```python
from build123d import *

# Parameters (mm, degrees)
SKETCH_W                           = 102
SKETCH_H                           = 105
SKETCH_R                           = 11
SKETCH_R_2                         = 13.5
PAD_DEPTH                          = 20
SKETCH001_W                        = 102
SKETCH001_H                        = 55
POCKET_DEPTH                       = 10
SKETCH002_W                        = 42
SKETCH002_H                        = 42
POCKET001_DEPTH                    = 16
POCKET002_DEPTH                    = 315.493809
POCKET002_LINEARPATTERN_2_DEPTH    = 315.493809
POCKET002_LINEARPATTERN_3_DEPTH    = 315.493809
POCKET002_LINEARPATTERN_4_DEPTH    = 315.493809
LINEARPATTERN001_COUNT             = 2
LINEARPATTERN001_PITCH             = 30
SKETCH004_R                        = 1.6
POCKET003_DEPTH                    = 4.001
CHAMFER_SIZE                       = 5
CHAMFER001_SIZE                    = 10
FILLET_R                           = 20
SKETCH006_R                        = 16
POCKET004_DEPTH                    = 16
SKETCH007_R                        = 3
POCKET005_DEPTH                    = 2
POCKET006_DEPTH                    = 4.001
SKETCH009_W                        = 4
SKETCH009_H                        = 42
POCKET007_DEPTH                    = 16
POCKET008_DEPTH                    = 2
POCKET009_DEPTH                    = 20.001
SKETCH012_R                        = 6.5
POCKET010_DEPTH                    = 8
SKETCH012_LINEARPATTERN002_2_R     = 6.5
POCKET010_LINEARPATTERN002_2_DEPTH = 8
SKETCH012_LINEARPATTERN002_3_R     = 6.5
POCKET010_LINEARPATTERN002_3_DEPTH = 8
LINEARPATTERN003_COUNT             = 3
LINEARPATTERN003_PITCH             = 15


with BuildPart() as part:
    # Sketch → Pad (new body)
    with BuildSketch(Plane.XY):
        with Locations((-14, -27.5)):
            Rectangle(SKETCH_W, SKETCH_H)
        with Locations((2, 0)):
            Circle(SKETCH_R, mode=Mode.SUBTRACT)
        with Locations((-40, 0)):
            Circle(SKETCH_R_2, mode=Mode.SUBTRACT)
    extrude(amount=PAD_DEPTH)

    # Sketch001 (on Face8 of Pad) → Pocket (cut)
    with BuildSketch(Plane.XY.offset(20)):
        with Locations((-14, -52.5)):
            Rectangle(SKETCH001_W, SKETCH001_H)
    extrude(amount=-POCKET_DEPTH, mode=Mode.SUBTRACT)

    # Sketch002 (on Face2 of Pocket) → Pocket001 (cut)
    with BuildSketch(Plane(origin=(0, 0, 0), x_dir=(1, 0, 0), z_dir=(0, 0, -1))):
        with Locations((2, 0)):
            Rectangle(SKETCH002_W, SKETCH002_H)
    extrude(amount=-POCKET001_DEPTH, mode=Mode.SUBTRACT)

    # Sketch003 (on Face2 of Pocket001) → Pocket002 (cut, through all)
    with BuildSketch(Plane(origin=(0, 0, 0), x_dir=(1, 0, 0), z_dir=(0, 0, -1))):
        with BuildLine():
            ThreePointArc((26, 35), (28, 33), (30, 35))
            Line((30, 35), (30, 45))
            ThreePointArc((30, 45), (28, 47), (26, 45))
            Line((26, 35), (26, 45))
        make_face()
    pocket002 = extrude(amount=-POCKET002_DEPTH, mode=Mode.SUBTRACT)

    # Sketch003 LinearPattern 2 → Pocket002 LinearPattern 2 (cut, through all)
    with BuildSketch(Plane(origin=(-28, 0, 0), x_dir=(1, 0, 0), z_dir=(0, 0, -1))):
        with BuildLine():
            ThreePointArc((26, 35), (28, 33), (30, 35))
            Line((30, 35), (30, 45))
            ThreePointArc((30, 45), (28, 47), (26, 45))
            Line((26, 35), (26, 45))
        make_face()
    pocket002_linearpattern_2 = extrude(amount=-POCKET002_LINEARPATTERN_2_DEPTH, mode=Mode.SUBTRACT)

    # Sketch003 LinearPattern 3 → Pocket002 LinearPattern 3 (cut, through all)
    with BuildSketch(Plane(origin=(-56, 0, 0), x_dir=(1, 0, 0), z_dir=(0, 0, -1))):
        with BuildLine():
            ThreePointArc((26, 35), (28, 33), (30, 35))
            Line((30, 35), (30, 45))
            ThreePointArc((30, 45), (28, 47), (26, 45))
            Line((26, 35), (26, 45))
        make_face()
    pocket002_linearpattern_3 = extrude(amount=-POCKET002_LINEARPATTERN_3_DEPTH, mode=Mode.SUBTRACT)

    # Sketch003 LinearPattern 4 → Pocket002 LinearPattern 4 (cut, through all)
    with BuildSketch(Plane(origin=(-84, 0, 0), x_dir=(1, 0, 0), z_dir=(0, 0, -1))):
        with BuildLine():
            ThreePointArc((26, 35), (28, 33), (30, 35))
            Line((30, 35), (30, 45))
            ThreePointArc((30, 45), (28, 47), (26, 45))
            Line((26, 35), (26, 45))
        make_face()
    pocket002_linearpattern_4 = extrude(amount=-POCKET002_LINEARPATTERN_4_DEPTH, mode=Mode.SUBTRACT)

    # LinearPattern001: Pocket002, Pocket002 LinearPattern 2, Pocket002 LinearPattern 3, Pocket002 LinearPattern 4 ×2
    with Locations(*[(0, -i * LINEARPATTERN001_PITCH, 0) for i in range(1, LINEARPATTERN001_COUNT)]):
        add(pocket002, mode=Mode.SUBTRACT)
        add(pocket002_linearpattern_2, mode=Mode.SUBTRACT)
        add(pocket002_linearpattern_3, mode=Mode.SUBTRACT)
        add(pocket002_linearpattern_4, mode=Mode.SUBTRACT)

    # Sketch004 (on Face46 of MultiTransform) → Pocket003 (cut, through all)
    with BuildSketch(Plane(origin=(0, 0, 16), x_dir=(1, 0, 0), z_dir=(0, 0, -1))):
        with Locations((16.5, 15.5)):
            Circle(SKETCH004_R)
        with Locations((16.5, -15.5)):
            Circle(SKETCH004_R)
        with Locations((-14.5, -15.5)):
            Circle(SKETCH004_R)
        with Locations((-14.5, 15.5)):
            Circle(SKETCH004_R)
    extrude(amount=-POCKET003_DEPTH, mode=Mode.SUBTRACT)

    # Chamfer
    chamfer_edges = [part.edges().sort_by_distance(p)[0] for p in [
        (-65, -80, 5),
        (37, -80, 5),
    ]]
    chamfer(chamfer_edges, length=CHAMFER_SIZE)

    # Chamfer001
    chamfer001_edges = [part.edges().sort_by_distance(p)[0] for p in [
        (37, -25, 15),
        (37, 25, 10),
        (-65, -25, 15),
    ]]
    chamfer(chamfer001_edges, length=CHAMFER001_SIZE)

    # Fillet
    fillet_edges = [part.edges().sort_by_distance(p)[0] for p in [
        (-65, 25, 10),
    ]]
    fillet(fillet_edges, radius=FILLET_R)

    # Sketch006 (on Face47 of Fillet) → Pocket004 (cut)
    with BuildSketch(Plane.XY.offset(20)):
        with Locations((-40, 0)):
            Circle(SKETCH006_R)
    extrude(amount=-POCKET004_DEPTH, mode=Mode.SUBTRACT)

    # Sketch007 (on Face47 of Pocket004) → Pocket005 (cut)
    with BuildSketch(Plane.XY.offset(20)):
        with Locations((16.5, 15.5)):
            Circle(SKETCH007_R)
        with Locations((-14.5, 15.5)):
            Circle(SKETCH007_R)
        with Locations((-14.5, -15.5)):
            Circle(SKETCH007_R)
        with Locations((16.5, -15.5)):
            Circle(SKETCH007_R)
    extrude(amount=-POCKET005_DEPTH, mode=Mode.SUBTRACT)

    # Sketch008 (on Face52 of Pocket005) → Pocket006 (cut, through all)
    with BuildSketch(Plane(origin=(0, 0, 16), x_dir=(1, 0, 0), z_dir=(0, 0, -1))):
        with BuildLine():
            ThreePointArc((-14.5, -17.1), (-12.9, -15.5), (-14.5, -13.9))
            Line((-14.5, -13.9), (-16.5, -13.9))
            ThreePointArc((-16.5, -13.9), (-18.1, -15.5), (-16.5, -17.1))
            Line((-14.5, -17.1), (-16.5, -17.1))
        make_face()
        with BuildLine():
            ThreePointArc((-14.5, 13.9), (-12.9, 15.5), (-14.5, 17.1))
            Line((-14.5, 17.1), (-16.5, 17.1))
            ThreePointArc((-16.5, 17.1), (-18.1, 15.5), (-16.5, 13.9))
            Line((-14.5, 13.9), (-16.5, 13.9))
        make_face()
        with BuildLine():
            ThreePointArc((16.5, 13.9), (18.1, 15.5), (16.5, 17.1))
            Line((16.5, 17.1), (14.5, 17.1))
            ThreePointArc((14.5, 17.1), (12.9, 15.5), (14.5, 13.9))
            Line((16.5, 13.9), (14.5, 13.9))
        make_face()
        with BuildLine():
            ThreePointArc((16.5, -17.1), (18.1, -15.5), (16.5, -13.9))
            Line((16.5, -13.9), (14.5, -13.9))
            ThreePointArc((14.5, -13.9), (12.9, -15.5), (14.5, -17.1))
            Line((16.5, -17.1), (14.5, -17.1))
        make_face()
    extrude(amount=-POCKET006_DEPTH, mode=Mode.SUBTRACT)

    # Sketch009 (on Face1 of Pocket006) → Pocket007 (cut)
    with BuildSketch(Plane(origin=(0, 0, 0), x_dir=(1, 0, 0), z_dir=(0, 0, -1))):
        with Locations((-21, 0)):
            Rectangle(SKETCH009_W, SKETCH009_H)
    extrude(amount=-POCKET007_DEPTH, mode=Mode.SUBTRACT)

    # Sketch010 (on Face49 of Pocket007) → Pocket008 (cut)
    with BuildSketch(Plane.XY.offset(20)):
        with BuildLine():
            ThreePointArc((-14.5, 12.5), (-11.5, 15.5), (-14.5, 18.5))
            Line((-14.5, 18.5), (-16.5, 18.5))
            ThreePointArc((-16.5, 18.5), (-19.5, 15.5), (-16.5, 12.5))
            Line((-14.5, 12.5), (-16.5, 12.5))
        make_face()
        with BuildLine():
            ThreePointArc((16.5, 12.5), (19.5, 15.5), (16.5, 18.5))
            Line((16.5, 18.5), (14.5, 18.5))
            ThreePointArc((14.5, 18.5), (11.5, 15.5), (14.5, 12.5))
            Line((16.5, 12.5), (14.5, 12.5))
        make_face()
        with BuildLine():
            ThreePointArc((16.5, -18.5), (19.5, -15.5), (16.5, -12.5))
            Line((16.5, -12.5), (14.5, -12.5))
            ThreePointArc((14.5, -12.5), (11.5, -15.5), (14.5, -18.5))
            Line((16.5, -18.5), (14.5, -18.5))
        make_face()
        with BuildLine():
            ThreePointArc((-14.5, -18.5), (-11.5, -15.5), (-14.5, -12.5))
            Line((-14.5, -12.5), (-16.5, -12.5))
            ThreePointArc((-16.5, -12.5), (-19.5, -15.5), (-16.5, -18.5))
            Line((-14.5, -18.5), (-16.5, -18.5))
        make_face()
    extrude(amount=-POCKET008_DEPTH, mode=Mode.SUBTRACT)

    # Sketch011 (on Face49 of Pocket008) → Pocket009 (cut, through all)
    with BuildSketch(Plane.XY.offset(20)):
        with BuildLine():
            ThreePointArc((0, -11), (11, 0), (0, 11))
            Line((0, 11), (-2, 11))
            ThreePointArc((-2, 11), (-13, 0), (-2, -11))
            Line((0, -11), (-2, -11))
        make_face()
    extrude(amount=-POCKET009_DEPTH, mode=Mode.SUBTRACT)

    # Sketch012 (on Face51 of Pocket009) → Pocket010 (cut)
    with BuildSketch(Plane.XY.offset(10)):
        with Locations((14, -65)):
            Circle(SKETCH012_R)
    pocket010 = extrude(amount=-POCKET010_DEPTH, mode=Mode.SUBTRACT)

    # Sketch012 LinearPattern002 2 → Pocket010 LinearPattern002 2 (cut)
    with BuildSketch(Plane(origin=(-28, 0, 10), x_dir=(1, 0, 0), z_dir=(0, 0, 1))):
        with Locations((14, -65)):
            Circle(SKETCH012_LINEARPATTERN002_2_R)
    pocket010_linearpattern002_2 = extrude(amount=-POCKET010_LINEARPATTERN002_2_DEPTH, mode=Mode.SUBTRACT)

    # Sketch012 LinearPattern002 3 → Pocket010 LinearPattern002 3 (cut)
    with BuildSketch(Plane(origin=(-56, 0, 10), x_dir=(1, 0, 0), z_dir=(0, 0, 1))):
        with Locations((14, -65)):
            Circle(SKETCH012_LINEARPATTERN002_3_R)
    pocket010_linearpattern002_3 = extrude(amount=-POCKET010_LINEARPATTERN002_3_DEPTH, mode=Mode.SUBTRACT)

    # LinearPattern003: Pocket010, Pocket010 LinearPattern002 2, Pocket010 LinearPattern002 3 ×3
    with Locations(*[(0, i * LINEARPATTERN003_PITCH, 0) for i in range(1, LINEARPATTERN003_COUNT)]):
        add(pocket010, mode=Mode.SUBTRACT)
        add(pocket010_linearpattern002_2, mode=Mode.SUBTRACT)
        add(pocket010_linearpattern002_3, mode=Mode.SUBTRACT)


solid = part.part
```
Check sheet for the modelled part. Datum: model origin and axes. Units: mm. A direction names the side the tool comes from. Coordinates: 2 decimals unless noted, no trailing zeros. Loops run counter-clockwise (first coordinate to the right, second up) from the corner with the lowest first, then second, coordinate; pieces in that order, holes last.
1) Access from +Z, -Z, +X, -X, +Y, -Y to the whole of each face (thin tool, end or side, straight path). Record for faces 1 (the face through (23, 0, 8)), 2 (the face through (19.5, 15.4, 19)), 3 (the face through (-56, -63, 5)).
2) Sectioned sample at B-B (x = -28). Record the boundary of the cut face in (y, z), and give its area (3 significant figures).
3) Sectioned sample at D-D (x = -42). Record the boundary of the cut face in (y, z).
4) Sectioned sample at A-A (y = 0). Record the boundary of the cut face in (x, z).
5) Material ranges on probe 1 along X at (y, z) = (0, 2.9); probe 2 along Y at (x, z) = (14, 4.5); probe 3 along Y at (x, z) = (-3, 6.75), recorded low to high.
6) Gauge pin test, flat ends, axial feed: pin 1 (4 mm diameter, centred on x = 13, y = -49, fed in from +Z); pin 2 (1.8 mm diameter, centred on x = 14.5, y = -14, fed in from +Z); pin 3 (8 mm diameter, centred on x = 12, z = 16.5, fed in from -Y); pin 4 (1.8 mm diameter, centred on x = -16, y = -16, fed in from +Z). Record the tip position at first contact, or that the pin passes through.
7) Release check for a two-part mould opening along X. For faces 4 (the face through (-2, -40, 5)), 5 (the face through (-62, -78, 5)), 6 (the face through (37, -21, 8)) record: released by +X, released by -X, zero draft, split by the parting line, or undercut.
8) Sectioned sample at C-C (z = 14). Record the boundary of the cut face in (x, y), and give its area (3 significant figures).
Check sheet entries:
1. face 1: -Z
1. face 2: +Z
1. face 3: +Z, -Z
2. outline: (-80, 0) - (-77, 0) - (-77, 10) - (-80, 10) - close; (-63, 0) - (-47, 0) - (-47, 10) - (-63, 10) - close; (-33, 0) - (-6.18, 0) - (-6.18, 4) - (-10.58, 4) - (-10.58, 20) - (-25, 20) - (-25, 10) - (-33, 10) - close; (6.18, 0) - (25, 0) - (25, 20) - (10.58, 20) - (10.58, 4) - (6.18, 4) - close
2. area: 882 mm2
3. outline: (-80, 0) - (-13.35, 0) - (-13.35, 4) - (-15.87, 4) - (-15.87, 20) - (-25, 20) - (-25, 10) - (-28.5, 10) - (-28.5, 2) - (-41.5, 2) - (-41.5, 10) - (-43.5, 10) - (-43.5, 2) - (-56.5, 2) - (-56.5, 10) - (-58.5, 10) - (-58.5, 2) - (-71.5, 2) - (-71.5, 10) - (-80, 10) - close; (13.35, 0) - (25, 0) - (25, 20) - (15.87, 20) - (15.87, 4) - (13.35, 4) - close
4. outline: (-65, 0) - (-53.5, 0) - (-53.5, 4) - (-56, 4) - (-56, 20) - (-65, 20) - close; (-26.5, 0) - (-23, 0) - (-23, 16) - (-13, 16) - (-13, 20) - (-24, 20) - (-24, 4) - (-26.5, 4) - close; (13, 16) - (23, 16) - (23, 0) - (37, 0) - (37, 20) - (13, 20) - close
5. probe 1: x = -65 to -53.5, -26.5 to -23, 23 to 37
5. probe 2: y = -80 to -71.5, -58.5 to -56.5, -43.5 to -41.5, -28.5 to -21, 21 to 25
5. probe 3: y = -80 to -21, 21 to 25
6. pin 1: stops at z = 2
6. pin 2: stops at z = 18
6. pin 3: stops at y = -25
6. pin 4: passes through
7. face 4: undercut
7. face 5: released by -X
7. face 6: released by +X
8. outline: (-65, -15) - (-55, -25) - (27, -25) - (37, -15) - (37, 15) - (27, 25) - (-45, 25) arc R20 ccw to (-65, 5) - close; hole circle Ø32 at (-40, 0); hole (-23, -21) - (23, -21) - (23, 21) - (-23, 21) - close
8. area: 2,130 mm2
